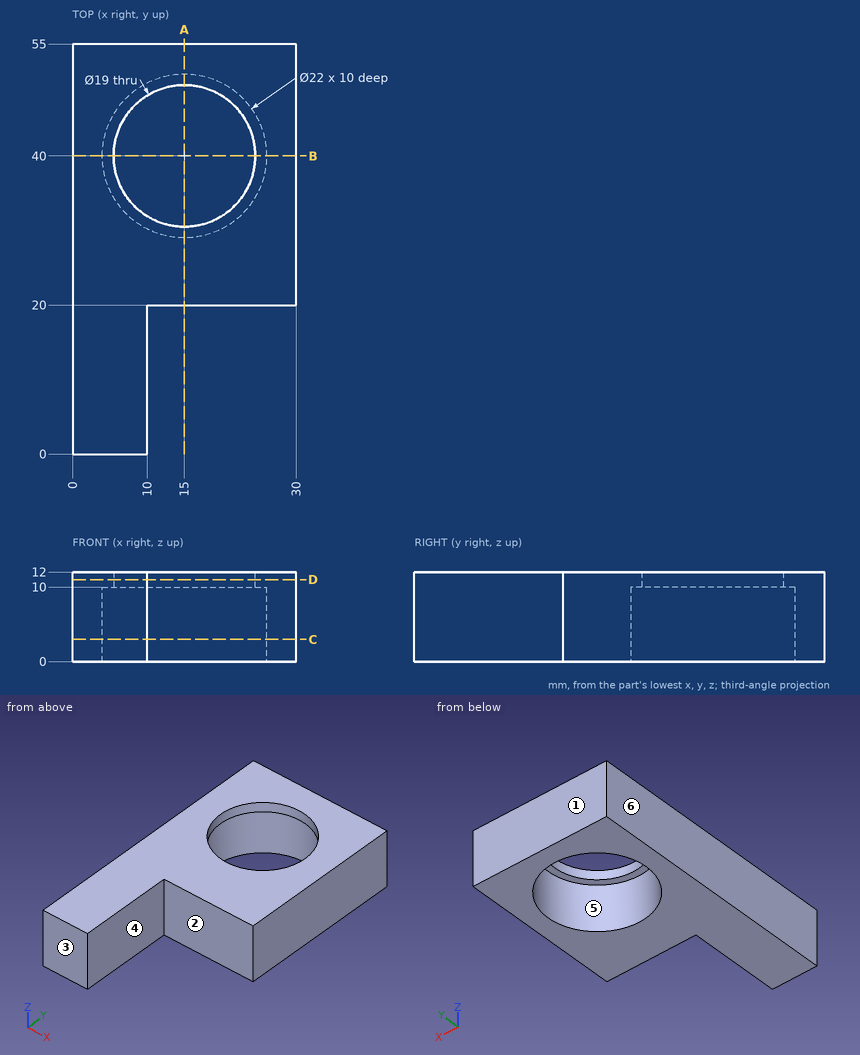
Input: dimensioned drawing with shaded views. Units: mm. Origin: part minimum x, y, z. A direction names the side the tool comes from. Coordinates: 2 decimals unless noted, no trailing zeros. Loops run counter-clockwise (first coordinate to the right, second up) from the corner with the lowest first, then second, coordinate; pieces in that order, holes last. Notation, with made-up numbers: M -3,78 L 42,78 A13 ccw 42,96 Z; hole C -7,-32 d11. An arc over 180 degrees is marked long. Use a Markdown table: item, result. Add a question column.
1) Section D-D, the plane z = 11. Return the cut outline in (x, y).
2) Section A-A, the plane x = 15. Return the cut outline in (y, z), plus the area to 3 significant figures.
3) Line query: L1, parallel to Y at x = 15, z = 4.25; L2, parallel to Y at x = 15, z = 10.5; L3, parallel to X at y = 40, z = 10.4. Output: solid intervals per line, ascending. Write a range as from..to.
4) Section C-C, the plane z = 3. Return the cut outline in (x, y).
5) Pin query (flat end, axial travel): P1, Ø4, axis at x = 13, z = 5, coming from the -Y side; P2, Ø1.5, axis at y = 8.5, z = 1.5, coming from the +X side. Return the tip coordinate at first contact, or that it passes through.
6) Set-up query: the marked faces 1 and 2. Return all of +Z, -Z, +X, -X, +Y, -Y with unobstructed straight access to the full face (end or side cutting, diameter ignored); none if empty.
7) Draft query along X for the marked faces 3, 4, 5 and 6. Return one class per face: +X half, -X half, draft (parallel to the pull), parting line (faces both ways), or undercut.
8) Section B-B, the plane y = 40. Return the cut outline in (x, z).
Answer below:
| question | item | result |
|---|---|---|
| 1 | outline | M 0,0 L 10,0 L 10,20 L 30,20 L 30,55 L 0,55 Z; hole C 15,40 d19 |
| 2 | outline | M 20,0 L 29,0 L 29,10 L 30.5,10 L 30.5,12 L 20,12 Z; M 49.5,10 L 51,10 L 51,0 L 55,0 L 55,12 L 49.5,12 Z |
| 2 | area | 162 mm2 |
| 3 | L1 | 20..29, 51..55 |
| 3 | L2 | 20..30.5, 49.5..55 |
| 3 | L3 | 0..5.5, 24.5..30 |
| 4 | outline | M 0,0 L 10,0 L 10,20 L 30,20 L 30,55 L 0,55 Z; hole C 15,40 d22 |
| 5 | P1 | y = 20 |
| 5 | P2 | x = 10 |
| 6 | face 1 | +Z, -Z, +X, -X, +Y |
| 6 | face 2 | +Z, -Z, +X, -Y |
| 7 | face 3 | draft |
| 7 | face 4 | +X half |
| 7 | face 5 | undercut |
| 7 | face 6 | -X half |
| 8 | outline | M 0,0 L 4,0 L 4,10 L 5.5,10 L 5.5,12 L 0,12 Z; M 24.5,10 L 26,10 L 26,0 L 30,0 L 30,12 L 24.5,12 Z |
